The drawing under review shows one solid part. Ordinate dimensions are in mm from its lowest x, y, z. A direction names the side the tool comes from. Give positions to 0.01 mm unless a question says otherwise; leave off trailing zeros. Order: outer loops, then holes, each group sorted by start corner. A loop starts at its lowest first (then second) coordinate and runs counter-clockwise, first axis right, second up. Notation, with made-up numbers: (87, 17) - (127, 17) arc R16 ccw to (127, 46) - close; hole circle Ø7 at (75.25, 36.5). An arc over 180 degrees is marked (long way). Use CSV: the item, a comma, the result in double quotes.
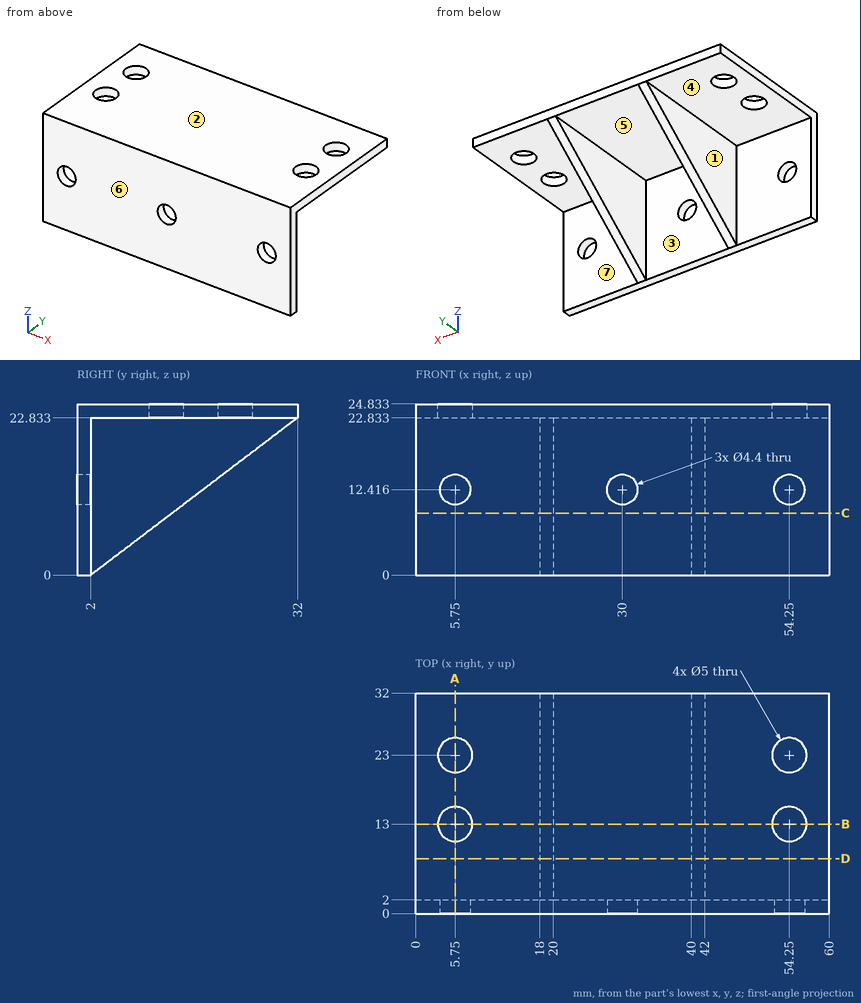
Item 1: Take a section at A-A, the plane x = 5.75. Give the boundary of the cut face in (y, z).
Results list:
outline,"(0, 0) - (2, 0) - (2, 10.22) - (0, 10.22) - close; (0, 14.62) - (2, 14.62) - (2, 22.83) - (10.5, 22.83) - (10.5, 24.83) - (0, 24.83) - close; (15.5, 22.83) - (20.5, 22.83) - (20.5, 24.83) - (15.5, 24.83) - close; (25.5, 22.83) - (32, 22.83) - (32, 24.83) - (25.5, 24.83) - close"
Item 2: Take a section at B-B, the plane y = 13. Give the boundary of the cut face in (x, z), and give its area (3 significant figures).
Results list:
outline,"(0, 22.83) - (3.25, 22.83) - (3.25, 24.83) - (0, 24.83) - close; (8.25, 22.83) - (18, 22.83) - (18, 8.37) - (20, 8.37) - (20, 22.83) - (40, 22.83) - (40, 8.37) - (42, 8.37) - (42, 22.83) - (51.75, 22.83) - (51.75, 24.83) - (8.25, 24.83) - close; (56.75, 22.83) - (60, 22.83) - (60, 24.83) - (56.75, 24.83) - close"
area,"158 mm2"
Item 3: Clearance check with flat-ended pins moving along their axes: pin 1 (12 mm diameter, centred on x = 40, z = 8.5, fed in from +Y); pin 2 (4.5 mm diameter, centred on x = 5.75, y = 13, fed in from +Z); pin 3 (16 mm diameter, centred on x = 28.5, y = 17.5, fed in from -Z); pin 4 (5.5 mm diameter, centred on x = 10.5, z = 13, fed in from +Y). State where each tip first meets the part, or that it passes through.
Results list:
pin 1,"stops at y = 21.05"
pin 2,"passes through"
pin 3,"stops at z = 22.83"
pin 4,"stops at y = 2"
Item 4: Wall thickness on L1, parallel to Y at x = 5.75, z = 23.65; L2, parallel to X at y = 25, z = 18.5; L3, parallel to Z at x = 48, y = 6.5: over which ranges is each line inside the solid? List them lowest first.
Results list:
L1,"y = 0 to 10.5, 15.5 to 20.5, 25.5 to 32"
L2,"x = 18 to 20, 40 to 42"
L3,"z = 22.83 to 24.83"
Item 5: Mouldability with a two-part tool opening along X and no side actions: class the marked faces 1, 2 and 3 as pulls with the +X half, pulls with the -X half, needs draft (parallel to the pull), parting line crosses it, or undercut.
Results list:
face 1,"pulls with the -X half"
face 2,"needs draft"
face 3,"undercut"
Item 6: Take a section at C-C, the plane z = 9. Give the boundary of the cut face in (x, y) (1 decimal), and give its area (3 significant figures).
Results list:
outline,"(0, 0) - (60, 0) - (60, 2) - (42, 2) - (42, 13.8) - (40, 13.8) - (40, 2) - (20, 2) - (20, 13.8) - (18, 13.8) - (18, 2) - (0, 2) - close"
area,"167 mm2"
Item 7: Tool access review of the marked faces 4, 5, 6 and 7: name each direction out of +Z, -Z, +X, -X, +Y, -Y from which nothing blocks a thin tool from reaching the whole face with its end or side.
Results list:
face 4,"-Z, -X, +Y"
face 5,"-Z, +Y"
face 6,"+Z, -Z, +X, -X, -Y"
face 7,"-Z, +X, +Y"
Item 8: Take a section at D-D, the plane y = 8. Give the boundary of the cut face in (x, z).
Results list:
outline,"(0, 22.83) - (18, 22.83) - (18, 4.57) - (20, 4.57) - (20, 22.83) - (40, 22.83) - (40, 4.57) - (42, 4.57) - (42, 22.83) - (60, 22.83) - (60, 24.83) - (0, 24.83) - close"
